Model file for the job. Use its own axes, mm. Face numbers are marked on the shaded views. A direction names the side the tool comes from. Give positions to 0.01 mm unless a question says otherwise; leave off trailing zeros. Loops run counter-clockwise (first coordinate to the right, second up) from the corner with the lowest first, then second, coordinate; pieces in that order, holes last. Notation, with made-up numbers: M 22.25,-9 L 67.25,-9 A12 ccw 67.25,9 Z; hole C 88.5,89 d3. An arc over 180 degrees is marked long. Use CSV: the item, a comma, the result in double quotes. Start each with the question number.
(1) Flat gauge pin, fed straight in: P1, Ø5.5, axis at y = 0, z = 0, coming from the +X side. Where does the tip first touch, or does it go through?
(2) Wall check: line 1 along Z through (x, y) = (1.7, 0); line 2 along X through (y, z) = (-2, 7). Give the ranges that are in metal, low to high. Write a range as from..to.
(3) Slice it at D-D on x = 2.5. List the corners of the cut face in (y, z), and give its area (3 significant figures).
(4) Two-plate mould, pull along Y, no slides. Class the marked faces 1, 2 and 3: pulls with the +Y half, pulls with the -Y half, needs draft (parallel to the pull), parting line crosses it, or undercut.
(5) Tool access for the marked faces 4 and 5: list every direction of +Z, -Z, +X, -X, +Y, -Y with a clear straight run to the whole face (end or side of a thin tool).
(6) Slice it at A-A on z = 0. List the corners of the cut face in (x, y), and give its area (3 significant figures).
(7) Slice it at C-C on x = 0.95. List the corners of the cut face in (y, z), and give its area (3 significant figures).
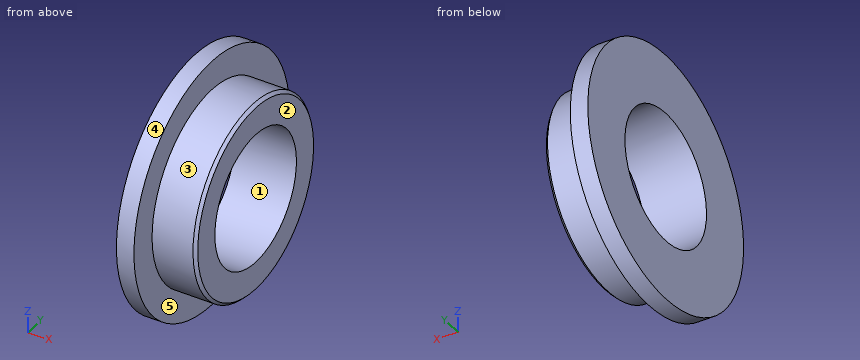
Solid Edge part; units mm, degrees
sketch "Sketch1" plane through (0, 0, 0) normal (0, -1, 0) x (1, 0, 0)
  line L0 (4.2, 4.5) -> (0, 4.5)
  line L1 (0, 4.5) -> (0, 8.59)
  line L2 (0, 8.59) -> (1.2, 8.59)
  line L3 (1.2, 8.59) -> (1.2, 6.59)
  line L4 (1.2, 6.59) -> (4.2, 6.59)
  line L5 (4.2, 6.59) -> (4.2, 4.5)
revolve "RevolvedProtrusion1" add sketch "Sketch1" angle 360 about axis through (0, 0, 0) along (1, 0, 0)
chamfer "Chamfer1" distance 0.2 angle 45 1 edges at (4.2, 0, -6.59)
Reply:
1,P1,"passes through"
2,line 1,"z = -6.59..-4.5, 4.5..6.59"
2,line 2,"x = 0..1.2"
3,outline,"C 0,0 d13.18; hole C 0,0 d9"
3,area,"72.8 mm^2"
4,face 1,"undercut"
4,face 2,"needs draft"
4,face 3,"parting line crosses it"
5,face 4,"+X, -X"
5,face 5,"+X"
6,outline,"M 0,-8.59 L 1.2,-8.59 L 1.2,-6.59 L 4,-6.59 L 4.2,-6.39 L 4.2,-4.5 L 0,-4.5 Z; M 0,4.5 L 4.2,4.5 L 4.2,6.39 L 4,6.59 L 1.2,6.59 L 1.2,8.59 L 0,8.59 Z"
6,area,"22.3 mm^2"
7,outline,"C 0,0 d17.18; hole C 0,0 d9"
7,area,"168 mm^2"
